The model under review builds one solid part; all positions refer to its coordinate system, in mm. Round coordinates to 2 decimals unless told otherwise and drop trailing zeros. Loops run counter-clockwise (first coordinate to the right, second up) from the corner with the lowest first, then second, coordinate; pieces in that order, holes last. Notation, with made-up numbers: M 3.25,63 L 38.25,63 A23 cw 38.25,101 Z; hole C -10,17.25 d5. An arc over 180 degrees is marked long. Answer in a Markdown table with one row per item. Add a question column.
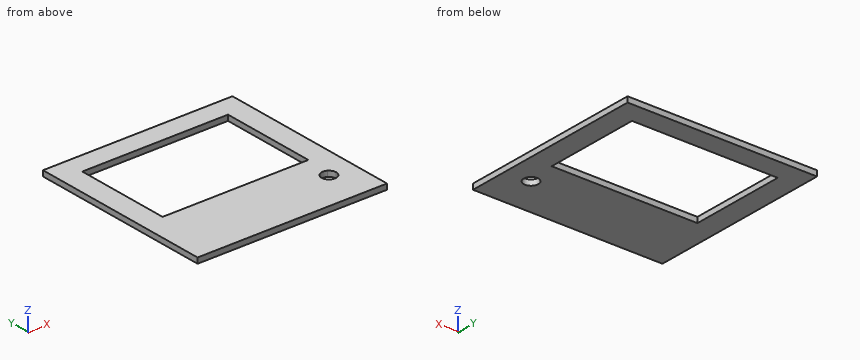
from build123d import *

# Parameters (mm, degrees)
F1_DEPTH = 3
F4_DEPTH = 25


with BuildPart() as f1:
    # F0 (on Top) → F1 (new body)
    with BuildSketch(Plane.XY):
        Polygon((40, 0), (40, -26.5), (0, -26.5), (0, -64), (52, -64), (52, 0), align=None)
        Polygon((40, 26.5), (40, 0), (52, 0), (52, 38), (0, 38), (0, 26.5), align=None)
    extrude(amount=F1_DEPTH)

    # F2: F1 across plane


with BuildPart() as f1_1:
    add(f1.part)
    add(f1.part.mirror(Plane.YZ))


with BuildPart() as f4:
    # F3 (on Top) → F4 (new body)
    with BuildSketch(Plane.XY):
        with BuildLine():
            ThreePointArc((40, -39.035898), (34.535898, -44.5), (42, -42.5))
            ThreePointArc((42, -42.5), (41.464102, -40.5), (40, -39.035898))
        make_face()
    extrude(amount=F4_DEPTH)


with BuildPart() as f1_2:
    add(f1_1.part)

    # F5: cut F4
    add(f4.part, mode=Mode.SUBTRACT)


solid = f1_2.part
1. Take a section at D-D, the plane x = 38. State the section outline as (y, z) points.
2. Take a section at B-B, the plane y = -11.5. State the section outline as (x, z) points.
3. Take a section at A-A, the plane z = 0.9. State the section outline as (x, y) points.
4. Take a section at C-C, the plane x = -34. State the section outline as (y, z) points, and give its area (3 significant figures).
5. To check wall thickness, follow probe 1 along Y at (x, z) = (38, 2.4); probe 2 along Y at (x, z) = (24, 1.7); probe 3 along X at (y, z) = (3, 1.7). State the ranges of each line that lie inside material, in increasing order.
Check sheet entries:
| question | item | result |
|---|---|---|
| 1 | outline | M -64,0 L -46.5,0 L -46.5,3 L -64,3 Z; M -38.5,0 L -26.5,0 L -26.5,3 L -38.5,3 Z; M 26.5,0 L 38,0 L 38,3 L 26.5,3 Z |
| 2 | outline | M -52,0 L -40,0 L -40,3 L -52,3 Z; M 40,0 L 52,0 L 52,3 L 40,3 Z |
| 3 | outline | M -52,-64 L 52,-64 L 52,38 L -52,38 Z; hole M -40,-26.5 L 40,-26.5 L 40,26.5 L -40,26.5 Z; hole M 40,-39.04 A4 ccw long 42,-42.5 A4 ccw Z |
| 4 | outline | M -64,0 L -26.5,0 L -26.5,3 L -64,3 Z; M 26.5,0 L 38,0 L 38,3 L 26.5,3 Z |
| 4 | area | 147 mm^2 |
| 5 | probe 1 | y = -64 to -46.5, -38.5 to -26.5, 26.5 to 38 |
| 5 | probe 2 | y = -64 to -26.5, 26.5 to 38 |
| 5 | probe 3 | x = -52 to -40, 40 to 52 |
